Could you check a few things on this model? Use its own coordinates, in mm. Give positions to 0.01 mm unless a question says otherwise; leave off trailing zeros. Loops run counter-clockwise (first coordinate to the right, second up) from the corner with the lowest first, then second, coordinate; pieces in that order, holes last. Notation, with made-up numbers: (65.5, -19.75) - (80.5, -19.75) arc R30 ccw to (80.5, 15.25) - close; hole circle Ø10 at (73.5, 88). An arc over 180 degrees is marked (long way). One line per item, written item: value. Start each with the question number.
Q1. If I drill on line 1 (Z direction, x = -63.5, y = 2.5) (3 decimals); line 2 (X direction, y = 0.9, z = -660.4) (3 decimals); line 3 (X direction, y = 2.15, z = -698.5) (3 decimals), over which ranges is the centre line in solid material (lowest first)? Write a range as from..to.
Q2. I'm going to push flat-ended pins straight in: P1, Ø5, axis at x = -188, z = -206.5, coming from the -Y side; P2, Ø1, axis at y = 1.5, z = -99.5, coming from the -X side; P3, Ø1.6, axis at y = 1, z = -612.5, coming from the +X side. Where does each tip first touch, or does it pass through?
Q3. I want a section at A-A (y = 1.2). Count the separate pieces of the cut face and the enclosed holes in it, then the cut area to 3 significant figures.
Q4. I want a section at B-B (z = -302). Please give me the cut outline in (x, y) (3 decimals).
Autodesk Inventor part; units mm, degrees
ref_plane "YZ Plane" through (0, 0, 0) normal (1, 0, 0) x (0, 1, 0)
ref_plane "XZ Plane" through (0, 0, 0) normal (0, 1, 0) x (-1, 0, 0)
ref_plane "XY Plane" through (0, 0, 0) normal (0, 0, 1) x (1, 0, 0)
sketch "Sketch1" plane through (0, 0, 0) normal (0, 1, 0) x (-1, 0, 0)
  line L0 (0, 0) -> (558.8, 0) construction
  line L1 (558.8, 0) -> (558.8, -711.2) construction
  line L2 (558.8, -711.2) -> (0, -711.2) construction
  line L3 (0, -711.2) -> (0, 0) construction
  line L4 (558.8, -355.6) -> (457.2, -355.6) construction
  line L5 (457.2, -355.6) -> (457.2, -425.45) construction
  line L6 (457.2, -425.45) -> (558.8, -425.45) construction
  line L7 (558.8, -425.45) -> (558.8, -355.6) construction
  line L8 (558.8, -355.6) -> (457.2, -355.6) construction
  line L9 (457.2, -355.6) -> (457.2, -285.75) construction
  line L10 (457.2, -285.75) -> (558.8, -285.75) construction
  line L11 (558.8, -285.75) -> (558.8, -355.6) construction
  line L12 (0, -355.6) -> (101.6, -355.6) construction
  line L13 (101.6, -355.6) -> (101.6, -425.45) construction
  line L14 (101.6, -425.45) -> (0, -425.45) construction
  line L15 (0, -425.45) -> (0, -355.6) construction
  line L16 (0, -355.6) -> (101.6, -355.6) construction
  line L17 (101.6, -355.6) -> (101.6, -285.75) construction
  line L18 (101.6, -285.75) -> (0, -285.75) construction
  line L19 (0, -285.75) -> (0, -355.6) construction
  line L20 (558.8, 0) -> (558.8, -57.15) construction
  line L21 (558.8, -57.15) -> (520.7, -57.15) construction
  line L22 (520.7, -57.15) -> (520.7, -120.65) construction
  line L23 (520.7, -120.65) -> (558.8, -120.65) construction
  line L24 (558.8, -120.65) -> (558.8, -57.15) construction
  line L25 (0, 0) -> (0, -57.15) construction
  line L26 (0, -57.15) -> (38.1, -57.15) construction
  line L27 (38.1, -57.15) -> (38.1, -120.65) construction
  line L28 (38.1, -120.65) -> (0, -120.65) construction
  line L29 (0, -120.65) -> (0, -57.15) construction
  line L30 (0, -711.2) -> (0, -654.05) construction
  line L31 (0, -654.05) -> (38.1, -654.05) construction
  line L32 (38.1, -654.05) -> (38.1, -590.55) construction
  line L33 (38.1, -590.55) -> (0, -590.55) construction
  line L34 (0, -590.55) -> (0, -654.05) construction
  line L35 (558.8, -711.2) -> (558.8, -654.05) construction
  line L36 (558.8, -654.05) -> (520.7, -654.05) construction
  line L37 (520.7, -654.05) -> (520.7, -590.55) construction
  line L38 (520.7, -590.55) -> (558.8, -590.55) construction
  line L39 (558.8, -590.55) -> (558.8, -654.05) construction
  line L40 (0, 0) -> (558.8, 0)
  line L41 (558.8, 0) -> (558.8, -57.15)
  line L42 (558.8, -57.15) -> (520.7, -57.15)
  line L43 (520.7, -57.15) -> (520.7, -120.65)
  line L44 (520.7, -120.65) -> (558.8, -120.65)
  line L45 (558.8, -120.65) -> (558.8, -285.75)
  line L46 (558.8, -285.75) -> (457.2, -285.75)
  line L47 (457.2, -285.75) -> (457.2, -425.45)
  line L48 (457.2, -425.45) -> (558.8, -425.45)
  line L49 (558.8, -425.45) -> (558.8, -590.55)
  line L50 (558.8, -590.55) -> (520.7, -590.55)
  line L51 (520.7, -590.55) -> (520.7, -654.05)
  line L52 (520.7, -654.05) -> (558.8, -654.05)
  line L53 (558.8, -654.05) -> (558.8, -711.2)
  line L54 (558.8, -711.2) -> (0, -711.2)
  line L55 (0, -711.2) -> (0, -654.05)
  line L56 (0, -654.05) -> (38.1, -654.05)
  line L57 (38.1, -654.05) -> (38.1, -590.55)
  line L58 (38.1, -590.55) -> (0, -590.55)
  line L59 (0, -590.55) -> (0, -425.45)
  line L60 (0, -425.45) -> (101.6, -425.45)
  line L61 (101.6, -425.45) -> (101.6, -285.75)
  line L62 (101.6, -285.75) -> (0, -285.75)
  line L63 (0, -285.75) -> (0, -120.65)
  line L64 (0, -120.65) -> (38.1, -120.65)
  line L65 (38.1, -120.65) -> (38.1, -57.15)
  line L66 (38.1, -57.15) -> (0, -57.15)
  line L67 (0, -57.15) -> (0, 0)
  dimension "d0" = 558.8
  dimension "d1" = 711.2
  dimension "d2" = 101.6
  dimension "d3" = 69.85
  dimension "d4" = 101.6
  dimension "d5" = 69.85
  dimension "d6" = 101.6
  dimension "d7" = 69.85
  dimension "d8" = 101.6
  dimension "d9" = 69.85
  dimension "d10" = 57.15
  dimension "d11" = 38.1
  dimension "d12" = 63.5
  dimension "d13" = 57.15
  dimension "d14" = 38.1
  dimension "d15" = 63.5
  dimension "d16" = 57.15
  dimension "d17" = 38.1
  dimension "d18" = 63.5
  dimension "d19" = 57.15
  dimension "d20" = 38.1
  dimension "d21" = 63.5
extrude "Extrusion1" add sketch "Sketch1" along normal blind 3.175
sketch "Sketch2" plane through (0, 3.175, 0) normal (0, 1, 0) x (1, 0, 0)
  line L0 (-558.8, 0) -> (0, 0)
  line L1 (0, 0) -> (0, 57.15)
  line L2 (0, 57.15) -> (-38.1, 57.15)
  line L3 (-38.1, 57.15) -> (-38.1, 120.65)
  line L4 (-38.1, 120.65) -> (0, 120.65)
  line L5 (0, 120.65) -> (0, 285.75)
  line L6 (0, 285.75) -> (-101.6, 285.75)
  line L7 (-101.6, 285.75) -> (-101.6, 425.45)
  line L8 (-101.6, 425.45) -> (0, 425.45)
  line L9 (0, 425.45) -> (0, 590.55)
  line L10 (0, 590.55) -> (-38.1, 590.55)
  line L11 (-38.1, 590.55) -> (-38.1, 654.05)
  line L12 (-38.1, 654.05) -> (0, 654.05)
  line L13 (0, 654.05) -> (0, 711.2)
  line L14 (0, 711.2) -> (-558.8, 711.2)
  line L15 (-558.8, 711.2) -> (-558.8, 654.05)
  line L16 (-558.8, 654.05) -> (-520.7, 654.05)
  line L17 (-520.7, 654.05) -> (-520.7, 590.55)
  line L18 (-520.7, 590.55) -> (-558.8, 590.55)
  line L19 (-558.8, 590.55) -> (-558.8, 425.45)
  line L20 (-558.8, 425.45) -> (-457.2, 425.45)
  line L21 (-457.2, 425.45) -> (-457.2, 285.75)
  line L22 (-457.2, 285.75) -> (-558.8, 285.75)
  line L23 (-558.8, 285.75) -> (-558.8, 120.65)
  line L24 (-558.8, 120.65) -> (-520.7, 120.65)
  line L25 (-520.7, 120.65) -> (-520.7, 57.15)
  line L26 (-520.7, 57.15) -> (-558.8, 57.15)
  line L27 (-558.8, 57.15) -> (-558.8, 0)
  point P0 (-546.1, 38.1)
  point P1 (-546.1, 50.8)
  point P2 (-12.7, 38.1)
  point P3 (-12.7, 50.8)
  point P4 (-12.7, 673.1)
  point P5 (-12.7, 660.4)
  point P6 (-546.1, 673.1)
  point P7 (-546.1, 660.4)
  dimension "d24" = 12.7
  dimension "d25" = 12.7
  dimension "d26" = 50.8
  dimension "d27" = 38.1
  dimension "d28" = 12.7
  dimension "d29" = 12.7
  dimension "d30" = 38.1
  dimension "d31" = 50.8
  dimension "d32" = 50.8
  dimension "d33" = 38.1
  dimension "d34" = 38.1
  dimension "d35" = 50.8
  dimension "d36" = 12.7
  dimension "d37" = 12.7
  dimension "d38" = 12.7
  dimension "d39" = 12.7
hole "Hole1" at (-546.1, 3.175, -38.1) at (-546.1, 3.175, -50.8) at (-12.7, 3.175, -38.1) at (-12.7, 3.175, -50.8) at (-12.7, 3.175, -673.1) at (-12.7, 3.175, -660.4) at (-546.1, 3.175, -673.1) at (-546.1, 3.175, -660.4) direction (0, -1, 0) diameter 6.35 end through all
sketch "Sketch3" plane through (0, 0, 0) normal (0, -1, 0) x (1, 0, 0)
  circle A0 centre (-546.1, -673.1) radius 3.175
  circle A1 centre (-12.7, -673.1) radius 3.175
  circle A2 centre (-12.7, -38.1) radius 3.175
  circle A3 centre (-546.1, -38.1) radius 3.175
  circle A4 centre (-546.1, -50.8) radius 3.175
  circle A5 centre (-12.7, -50.8) radius 3.175
  circle A6 centre (-12.7, -660.4) radius 3.175
  circle A7 centre (-546.1, -660.4) radius 3.175
  line L0 (0, 0) -> (-558.8, 0)
  line L1 (-558.8, 0) -> (-558.8, -57.15)
  line L2 (-558.8, -57.15) -> (-520.7, -57.15)
  line L3 (-520.7, -57.15) -> (-520.7, -120.65)
  line L4 (-520.7, -120.65) -> (-558.8, -120.65)
  line L5 (-558.8, -120.65) -> (-558.8, -285.75)
  line L6 (-558.8, -285.75) -> (-457.2, -285.75)
  line L7 (-457.2, -285.75) -> (-457.2, -425.45)
  line L8 (-457.2, -425.45) -> (-558.8, -425.45)
  line L9 (-558.8, -425.45) -> (-558.8, -590.55)
  line L10 (-558.8, -590.55) -> (-520.7, -590.55)
  line L11 (-520.7, -590.55) -> (-520.7, -654.05)
  line L12 (-520.7, -654.05) -> (-558.8, -654.05)
  line L13 (-558.8, -654.05) -> (-558.8, -711.2)
  line L14 (-558.8, -711.2) -> (0, -711.2)
  line L15 (0, -711.2) -> (0, -654.05)
  line L16 (0, -654.05) -> (-38.1, -654.05)
  line L17 (-38.1, -654.05) -> (-38.1, -590.55)
  line L18 (-38.1, -590.55) -> (0, -590.55)
  line L19 (0, -590.55) -> (0, -425.45)
  line L20 (0, -425.45) -> (-101.6, -425.45)
  line L21 (-101.6, -425.45) -> (-101.6, -285.75)
  line L22 (-101.6, -285.75) -> (0, -285.75)
  line L23 (0, -285.75) -> (0, -120.65)
  line L24 (0, -120.65) -> (-38.1, -120.65)
  line L25 (-38.1, -120.65) -> (-38.1, -57.15)
  line L26 (-38.1, -57.15) -> (0, -57.15)
  line L27 (0, -57.15) -> (0, 0)
  point P0 (-12.7, -279.4)
  point P1 (-12.7, -203.2)
  point P2 (-12.7, -431.8)
  point P3 (-12.7, -508)
  point P4 (-546.1, -431.8)
  point P5 (-546.1, -508)
  point P6 (-546.1, -279.4)
  point P7 (-546.1, -203.2)
  dimension "d47" = 12.7
  dimension "d48" = 12.7
  dimension "d49" = 82.55
  dimension "d50" = 6.35
  dimension "d51" = 6.35
  dimension "d52" = 82.55
  dimension "d53" = 12.7
  dimension "d54" = 12.7
  dimension "d55" = 12.7
  dimension "d56" = 12.7
  dimension "d57" = 6.35
  dimension "d58" = 82.55
  dimension "d59" = 6.35
  dimension "d60" = 12.7
  dimension "d61" = 82.55
  dimension "d62" = 12.7
hole "Hole2" at (-12.7, 0, -279.4) at (-12.7, 0, -203.2) at (-12.7, 0, -431.8) at (-12.7, 0, -508) at (-546.1, 0, -431.8) at (-546.1, 0, -508) at (-546.1, 0, -279.4) at (-546.1, 0, -203.2) direction (0, 1, 0) diameter 6.35 end through all
sketch "Sketch4" plane through (0, 0, 0) normal (0, -1, 0) x (1, 0, 0)
  circle A0 centre (-546.1, -279.4) radius 3.175
  circle A1 centre (-546.1, -431.8) radius 3.175
  circle A2 centre (-12.7, -431.8) radius 3.175
  circle A3 centre (-12.7, -279.4) radius 3.175
  circle A4 centre (-12.7, -203.2) radius 3.175
  circle A5 centre (-12.7, -508) radius 3.175
  circle A6 centre (-546.1, -508) radius 3.175
  circle A7 centre (-546.1, -203.2) radius 3.175
  circle A8 centre (-546.1, -673.1) radius 3.175
  circle A9 centre (-12.7, -673.1) radius 3.175
  circle A10 centre (-12.7, -38.1) radius 3.175
  circle A11 centre (-546.1, -38.1) radius 3.175
  circle A12 centre (-546.1, -50.8) radius 3.175
  circle A13 centre (-12.7, -50.8) radius 3.175
  circle A14 centre (-12.7, -660.4) radius 3.175
  circle A15 centre (-546.1, -660.4) radius 3.175
  line L0 (0, 0) -> (-558.8, 0)
  line L1 (-558.8, 0) -> (-558.8, -57.15)
  line L2 (-558.8, -57.15) -> (-520.7, -57.15)
  line L3 (-520.7, -57.15) -> (-520.7, -120.65)
  line L4 (-520.7, -120.65) -> (-558.8, -120.65)
  line L5 (-558.8, -120.65) -> (-558.8, -285.75)
  line L6 (-558.8, -285.75) -> (-457.2, -285.75)
  line L7 (-457.2, -285.75) -> (-457.2, -425.45)
  line L8 (-457.2, -425.45) -> (-558.8, -425.45)
  line L9 (-558.8, -425.45) -> (-558.8, -590.55)
  line L10 (-558.8, -590.55) -> (-520.7, -590.55)
  line L11 (-520.7, -590.55) -> (-520.7, -654.05)
  line L12 (-520.7, -654.05) -> (-558.8, -654.05)
  line L13 (-558.8, -654.05) -> (-558.8, -711.2)
  line L14 (-558.8, -711.2) -> (0, -711.2)
  line L15 (0, -711.2) -> (0, -654.05)
  line L16 (0, -654.05) -> (-38.1, -654.05)
  line L17 (-38.1, -654.05) -> (-38.1, -590.55)
  line L18 (-38.1, -590.55) -> (0, -590.55)
  line L19 (0, -590.55) -> (0, -425.45)
  line L20 (0, -425.45) -> (-101.6, -425.45)
  line L21 (-101.6, -425.45) -> (-101.6, -285.75)
  line L22 (-101.6, -285.75) -> (0, -285.75)
  line L23 (0, -285.75) -> (0, -120.65)
  line L24 (0, -120.65) -> (-38.1, -120.65)
  line L25 (-38.1, -120.65) -> (-38.1, -57.15)
  line L26 (-38.1, -57.15) -> (0, -57.15)
  line L27 (0, -57.15) -> (0, 0)
  point P0 (-495.3, -698.5)
  point P1 (-368.3, -698.5)
  point P2 (-190.5, -698.5)
  point P3 (-63.5, -698.5)
  point P4 (-495.3, -12.7)
  point P5 (-368.3, -12.7)
  point P6 (-190.5, -12.7)
  point P7 (-63.5, -12.7)
  dimension "d70" = 63.5
  dimension "d71" = 12.7
  dimension "d72" = 12.7
  dimension "d73" = 190.5
  dimension "d74" = 63.5
  dimension "d75" = 12.7
  dimension "d76" = 12.7
  dimension "d77" = 190.5
  dimension "d78" = 12.7
  dimension "d79" = 63.5
  dimension "d80" = 12.7
  dimension "d81" = 190.5
  dimension "d82" = 63.5
  dimension "d83" = 12.7
  dimension "d84" = 12.7
  dimension "d85" = 190.5
hole "Hole3" at (-495.3, 0, -698.5) at (-368.3, 0, -698.5) at (-190.5, 0, -698.5) at (-63.5, 0, -698.5) at (-495.3, 0, -12.7) at (-368.3, 0, -12.7) at (-190.5, 0, -12.7) at (-63.5, 0, -12.7) direction (0, 1, 0) diameter 6.35 end through all
properties part number "base"
Worked answers:
1. line 1: z = -711.2..-701.675, -695.325..-425.45, -285.75..-15.875, -9.525..0
1. line 2: x = -558.8..-549.275, -542.925..-15.875, -9.525..0
1. line 3: x = -558.8..-498.475, -492.125..-371.475, -365.125..-193.675, -187.325..-66.675, -60.325..0
2. P1: stops at y = 0
2. P2: stops at x = -520.7
2. P3: stops at x = -38.1
3. separate pieces: 1
3. enclosed holes: 24
3. area: 359,000 mm²
4. outline: (-457.2, 0) - (-101.6, 0) - (-101.6, 3.175) - (-457.2, 3.175) - close
